The model under review builds one solid part; all positions refer to its coordinate system, in mm. A direction names the side the tool comes from. Round coordinates to 2 decimals unless told otherwise and drop trailing zeros. Order: outer loops, then holes, each group sorted by start corner. A loop starts at its lowest first (then second) coordinate and runs counter-clockwise, first axis right, second up. Notation, with made-up numbers: M 21,11 L 60,11 A19 cw 60,26 Z; hole C 68,41 d11. An arc over 180 degrees is marked long. Answer as a JSON object with one key per item and string values. Group by question number.
1) Consider section D-D, the plane y = -14. Write out the cut boundary in (x, z).
2) The part is to be moulded in two halves that separate along Z. For faces 1 (the cylindrical face through (19.66, 20.59, -4.15)), 2 (the cylindrical face through (19.66, -5.506, -24.796)), 3 (the flat face through (39.878, 5, -5)), say which applies: +Z half, -Z half, draft (parallel to the pull), parting line (faces both ways), or undercut.
3) Consider section B-B, the plane z = 19.05. Write out the cut boundary in (x, y), then the cut area to 3 significant figures.
4) Insertion check: pin 1 Ø1 at (y, z) = (-2, 16) entering from -X; pin 2 Ø3.5 at (x, y) = (11.5, 0.5) entering from +Z; pin 3 Ø8 at (x, y) = (16.5, -1.5) entering from -Z; pin 4 Ø8 at (x, y) = (30, 16.5) entering from +Z. Each pin has a flat end and moves straight along its axis. Give the tip position at first contact, or say it passes through.
5) For faces 4 (the flat face through (0, 5, -5)), 5 (the flat face through (20, 0, -6.35)), list the 3-axis set-ups (+Z, -Z, +X, -X, +Y, -Y) from which the entire face can be reached by the end or side of a thin tool; tool diameter is ignored.
6) Consider section A-A, the plane y = 0. Write out the cut boundary in (x, z).
7) To check wall thickness, follow line 1 (Z direction, x = 19.5, y = 0); line 2 (Y direction, x = 5.5, z = -3.5); line 3 (Y direction, x = 20, z = 11). State the ranges of each line that lie inside material, in increasing order.
8) Consider section C-C, the plane x = 35.5. Count the separate pieces of the cut face and the enclosed holes in it, then the cut area to 3 significant figures.
```python
from build123d import *

# Parameters (mm, degrees)
SKETCH2_R                  = 25.4
BOSS_EXTRUDE1_DEPTH        = 39.878
TAP_DRILL_FOR_10_32_TAP1_D = 4.0386


with BuildPart() as part:
    # Sketch2 → Boss-Extrude1 (new body)
    with BuildSketch(Plane.YZ):
        Circle(SKETCH2_R)
        Polygon((3.666174209, 6.35), (-3.666174209, 6.35), (-7.332348419, 0), (-3.666174209, -6.35), (3.666174209, -6.35), (7.332348419, 0), align=None, mode=Mode.SUBTRACT)
    extrude(amount=BOSS_EXTRUDE1_DEPTH)

    # Tap Drill for #10-32 Tap1 (through all)
    with Locations(Plane.YZ.offset(39.878)):
        with Locations((-14.893889741, 11.877480725), (0, 19.05), (14.893889741, 11.877480725), (18.572376727, -4.239023792), (8.26548523, -17.163456934), (-8.26548523, -17.163456934), (-18.572376727, -4.239023792)):
            Hole(TAP_DRILL_FOR_10_32_TAP1_D / 2)


solid = part.part
```
Results list:
{
 "1": {"outline": "M 0,-21.19 L 39.88,-21.19 L 39.88,10.07 L 0,10.07 Z; M 0,13.69 L 39.88,13.69 L 39.88,21.19 L 0,21.19 Z"},
 "2": {"face 1": "undercut", "face 2": "parting line", "face 3": "draft"},
 "3": {"outline": "M 0,-16.8 L 39.88,-16.8 L 39.88,-2.02 L 0,-2.02 Z; M 0,2.02 L 39.88,2.02 L 39.88,16.8 L 0,16.8 Z", "area": "1,180 mm^2"},
 "4": {"pin 1": "x = 0", "pin 2": "z = 25.4", "pin 3": "z = -25.4", "pin 4": "z = 22.11"},
 "5": {"face 4": "+Z, -Z, -X, +Y, -Y", "face 5": "+X, -X"},
 "6": {"outline": "M 0,-25.4 L 39.88,-25.4 L 39.88,-6.35 L 0,-6.35 Z; M 0,6.35 L 39.88,6.35 L 39.88,17.03 L 0,17.03 Z; M 0,21.07 L 39.88,21.07 L 39.88,25.4 L 0,25.4 Z"},
 "7": {"line 1": "-25.4 to -6.35, 6.35 to 17.03, 21.07 to 25.4", "line 2": "-25.16 to -20.45, -16.69 to -5.31, 5.31 to 16.69, 20.45 to 25.16", "line 3": "-22.89 to -16.71, -13.08 to 13.08, 16.71 to 22.89"},
 "8": {"separate pieces": "1", "enclosed holes": "8", "area": "1,800 mm^2"}
}
